```python
from build123d import *

# Parameters (mm, degrees)
BOSS_EXTRUDE1_DEPTH      = 2.5
BOSS_EXTRUDE1_DEPTH_BACK = 2.5
SKETCH2_W                = 30
SKETCH2_H                = 30
BOSS_EXTRUDE2_DEPTH      = 4
SKETCH3_R                = 1.135899117
CUT_EXTRUDE1_DEPTH       = 14.334397369
CUT_EXTRUDE1_DEPTH_BACK  = 5


with BuildPart() as part:
    # Sketch1 → Boss-Extrude1 (new body, two sides)
    with BuildSketch(Plane(origin=(0, 0, 0), x_dir=(1, 0, 0), z_dir=(0, 1, 0))) as boss_extrude1_sk:
        with BuildLine():
            Line((12.299846055, 27.042802031), (12.299846055, 15.43488972))
            add(Edge.make_bspline(
                [(12.299846055, 15.43488972), (30.534020994, -10.609424361), (-5.28178023, -16.186011799)],
                knots=[0, 0, 0, 1, 1, 1], degree=2))
            ThreePointArc((-5.28178023, -16.186011799), (-9.455741342, -21.893729502), (-3.748023639, -26.067690614))
            add(Edge.make_bspline(
                [(22.317047717, 18.444557689), (24.010987248, 15.756852788), (26.568030042, 10.329200416), (28.199135579, 4.70608307), (28.530980206, -0.219774719), (28.112095037, -4.221352146), (26.937580955, -8.124121484), (25.039004829, -11.720082951), (22.553291074, -14.857561986), (18.908458845, -18.15546642), (13.009520485, -21.610616265), (6.232054982, -23.983751971), (-0.197461384, -25.517985733), (-3.748023639, -26.067690614)],
                knots=[0.045025553, 0.045025553, 0.045025553, 0.134554407, 0.224083261, 0.313612116, 0.373298019, 0.432983922, 0.492669825, 0.552355728, 0.612041631, 0.701570485, 0.820942291, 0.910471146, 1, 1, 1], degree=2))
            ThreePointArc((22.317047717, 18.444557689), (17.956231252, 23.498367255), (12.299846055, 27.042802031))
        make_face()
    extrude(amount=BOSS_EXTRUDE1_DEPTH)
    extrude(boss_extrude1_sk.sketch, amount=-BOSS_EXTRUDE1_DEPTH_BACK)

    # Sketch2 → Boss-Extrude2 (add)
    with BuildSketch(Plane.ZY.offset(-12.299846055)):
        with Locations((-17.236867662, -0.834397369)):
            Rectangle(SKETCH2_W, SKETCH2_H)
    extrude(amount=BOSS_EXTRUDE2_DEPTH)

    # Sketch3 → Cut-Extrude1 (cut, two sides)
    with BuildSketch(Plane.XZ.offset(2.5)) as cut_extrude1_sk:
        with Locations((-5.323414867, 21.345746187)):
            Circle(SKETCH3_R)
    extrude(amount=CUT_EXTRUDE1_DEPTH, mode=Mode.SUBTRACT)
    extrude(cut_extrude1_sk.sketch, amount=-CUT_EXTRUDE1_DEPTH_BACK, mode=Mode.SUBTRACT)


solid = part.part
```
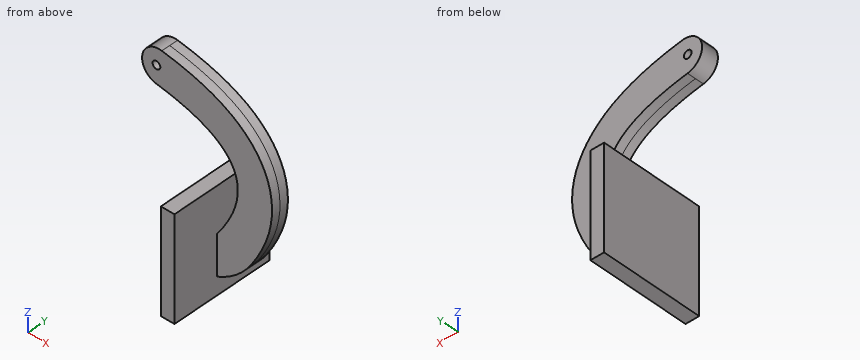
Build history of the part. All positions in model axes, mm. Coordinates: 2 decimals unless noted, no trailing zeros. Order: outer loops, then holes, each group sorted by start corner. A loop starts at its lowest first (then second) coordinate and runs counter-clockwise, first axis right, second up. Notation, with made-up numbers: (81, -14.5) -> (125, -14.5) arc R19 cw to (125, 18.5) -> close; hole circle Ø10 at (40, 48.25). An arc over 180 degrees is marked (long way). Answer in a Markdown table with one row per item. Add a question column.
Q1. Wall check: line 1 along Y through (x, z) = (1.5, 19.5); line 2 along X through (y, z) = (-4.5, -8); line 3 along Z through (x, y) = (-5, -0.25). Give the ranges that are in metal, low to high. Write a range as [from, to].
Q2. Band-saw the part on A-A, the plane y = -13.5. List the corners of the cut face in (x, z), then the cut area to 3 significant figures.
Q3. Drop flat-ended pins along their axis: pin 1 (4 mm diameter, centred on y = -10, z = -13, fed in from -X); pin 2 (5 mm diameter, centred on y = 9, z = -20.5, fed in from +X); pin 3 (10 mm diameter, centred on y = 7, z = -17, fed in from +X). Give the stop position or say it passes through.
Answers follow:
| question | item | result |
|---|---|---|
| 1 | line 1 | [-2.5, 2.5] |
| 1 | line 2 | [8.3, 12.3] |
| 1 | line 3 | [16.14, 20.26], [22.43, 26.1] |
| 2 | outline | (8.3, -32.24) -> (12.3, -32.24) -> (12.3, -2.24) -> (8.3, -2.24) -> close |
| 2 | area | 120 mm^2 |
| 3 | pin 1 | x = 8.3 |
| 3 | pin 2 | x = 12.3 |
| 3 | pin 3 | x = 24.41 |
